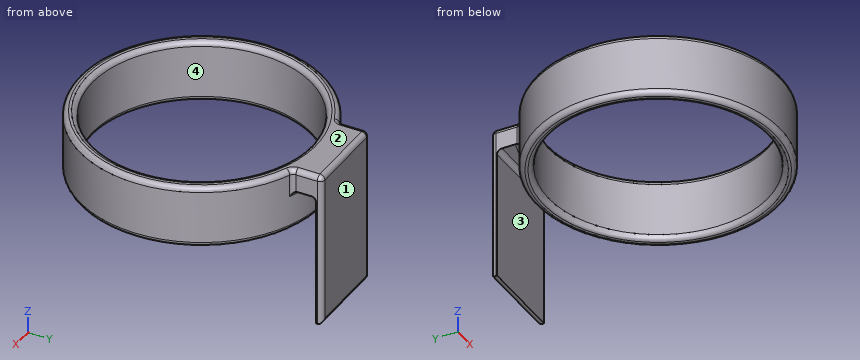
```python
from build123d import *

# Parameters (mm, degrees)
F0_R     = 49.53
F0_R_2   = 44.45
F1_DEPTH = 25.4
F3_DEPTH = 17.5
F4_R     = 2


with BuildPart() as f1:
    # F0 (on Top) → F1 (new body)
    with BuildSketch(Plane.XY):
        Circle(F0_R)
        Circle(F0_R_2, mode=Mode.SUBTRACT)
    extrude(amount=F1_DEPTH)

    # F2 (on Right) → F3 (join, symmetric)
    with BuildSketch(Plane.YZ):
        Polygon((58.382712847, 25.4), (45.682712847, 25.4), (45.682712847, 16.2404105067), (55.88, 16.2404105067), (55.88, -37.6108922064), (58.382712847, -38.1), align=None)
    extrude(amount=F3_DEPTH, both=True)

    # F4
    f4_edges = [f1.edges().sort_by_distance(p)[0] for p in [
        (0, 55.88, 16.240411),
        (0, 49.53, 16.240411),
        (17.5, 46.335417, 20.820205),
        (-17.5, 46.335417, 20.820205),
        (0, 58.382713, 25.4),
        (-44.45, 0, 25.4),
        (-49.53, 0, 0),
        (49.53, 0, 12.7),
        (-28.164214, -40.743072, 25.4),
        (40.743072, 28.164214, 25.4),
        (44.45, 0, 12.7),
        (-44.45, 0, 0),
        (-17.5, 58.382713, -6.35),
        (17.5, 58.382713, -6.35),
        (0, 58.382713, -38.1),
        (17.5, 52.359065, 25.4),
        (-17.5, 52.359065, 25.4),
    ]]
    fillet(f4_edges, radius=F4_R)


solid = f1.part
```
The listing builds one solid part. Answer for the finished solid, in the listing's coordinates (mm). Face numbers are marked on the shaded views. Round coordinates to 2 decimals unless told otherwise and drop trailing zeros. Loops run counter-clockwise (first coordinate to the right, second up) from the corner with the lowest first, then second, coordinate; pieces in that order, holes last.
1) Consider line 1 (Y direction, x = 0, z = 11.75); line 2 (Y direction, x = -16.5, z = 3.5); line 3 (Y direction, x = 1.5, z = -23). Determine where each line is inside the solid, lowest interval first.
Outcome:
line 1: y = -49.53 to -44.45, 44.45 to 49.53, 55.88 to 58.38
line 2: y = -46.7 to -41.27, 41.27 to 46.7, 55.88 to 58.11
line 3: y = 55.88 to 58.38
2) A cutting plane is placed at A-A on z = 5.5. Determine the outline of the cut face in (x, y), plus the area to 3 significant figures.
Outcome:
outline: circle Ø99.06 at (0, 0); (-17.5, 55.88) - (17.5, 55.88) - (17.5, 56.38) arc R2 ccw to (15.5, 58.38) - (-15.5, 58.38) arc R2 ccw to (-17.5, 56.38) - close; hole circle Ø88.9 at (0, 0)
area: 1,590 mm2
3) For a pull along Y with two mould halves and no side action, classify the marked faces 1, 2, 3 and 4 as released by +Y, released by -Y, zero draft, split by the parting line, or undercut.
Outcome:
face 1: released by +Y
face 2: zero draft
face 3: undercut
face 4: undercut
4) A cutting plane is placed at C-C on x = 0. Determine the outline of the cut face in (y, z), plus the area to 3 significant figures.
Outcome:
outline: (-49.53, 2) arc R2 ccw to (-47.53, 0) - (-46.45, 0) arc R2 ccw to (-44.45, 2) - (-44.45, 23.4) arc R2 ccw to (-46.45, 25.4) - (-47.53, 25.4) arc R2 ccw to (-49.53, 23.4) - close; (44.45, 2) arc R2 ccw to (46.45, 0) - (47.53, 0) arc R2 ccw to (49.53, 2) - (49.53, 14.24) arc R2 cw to (51.53, 16.24) - (53.88, 16.24) arc R2 cw to (55.88, 14.24) - (55.88, -37.61) - (56, -37.63) arc R2 ccw to (58.38, -35.67) - (58.38, 23.4) arc R2 ccw to (56.38, 25.4) - (46.45, 25.4) arc R2 ccw to (44.45, 23.4) - close
area: 468 mm2
5) Given P1, Ø8, axis at x = -38.5, z = -5, coming from the -Y side; P2, Ø8, axis at x = -32.5, z = 17.5, coming from the +Y side; P3, Ø6, axis at y = 12.5, z = -2, coming from the -X side; P4, Ø4.5, axis at x = 7.5, y = 50.5, coming from the -Z side, each flat-ended and moving along its own axis, determine where each tip first touches the part or whether it passes through.
Outcome:
P1: passes through
P2: stops at y = 40.51
P3: stops at x = -47.79
P4: stops at z = 0.46
6) A cutting plane is placed at D-D on z = -20.5. Determine the outline of the cut face in (x, y), plus the area to 3 significant figures.
Outcome:
outline: (-17.5, 55.88) - (17.5, 55.88) - (17.5, 56.38) arc R2 ccw to (15.5, 58.38) - (-15.5, 58.38) arc R2 ccw to (-17.5, 56.38) - close
area: 85.9 mm2
7) A cutting plane is placed at B-B on y = 0. Determine the outline of the cut face in (x, z), plus the area to 3 significant figures.
Outcome:
outline: (-49.53, 2) arc R2 ccw to (-47.53, 0) - (-46.45, 0) arc R2 ccw to (-44.45, 2) - (-44.45, 23.4) arc R2 ccw to (-46.45, 25.4) - (-47.53, 25.4) arc R2 ccw to (-49.53, 23.4) - close; (44.45, 2) arc R2 ccw to (46.45, 0) - (47.53, 0) arc R2 ccw to (49.53, 2) - (49.53, 23.4) arc R2 ccw to (47.53, 25.4) - (46.45, 25.4) arc R2 ccw to (44.45, 23.4) - close
area: 251 mm2
